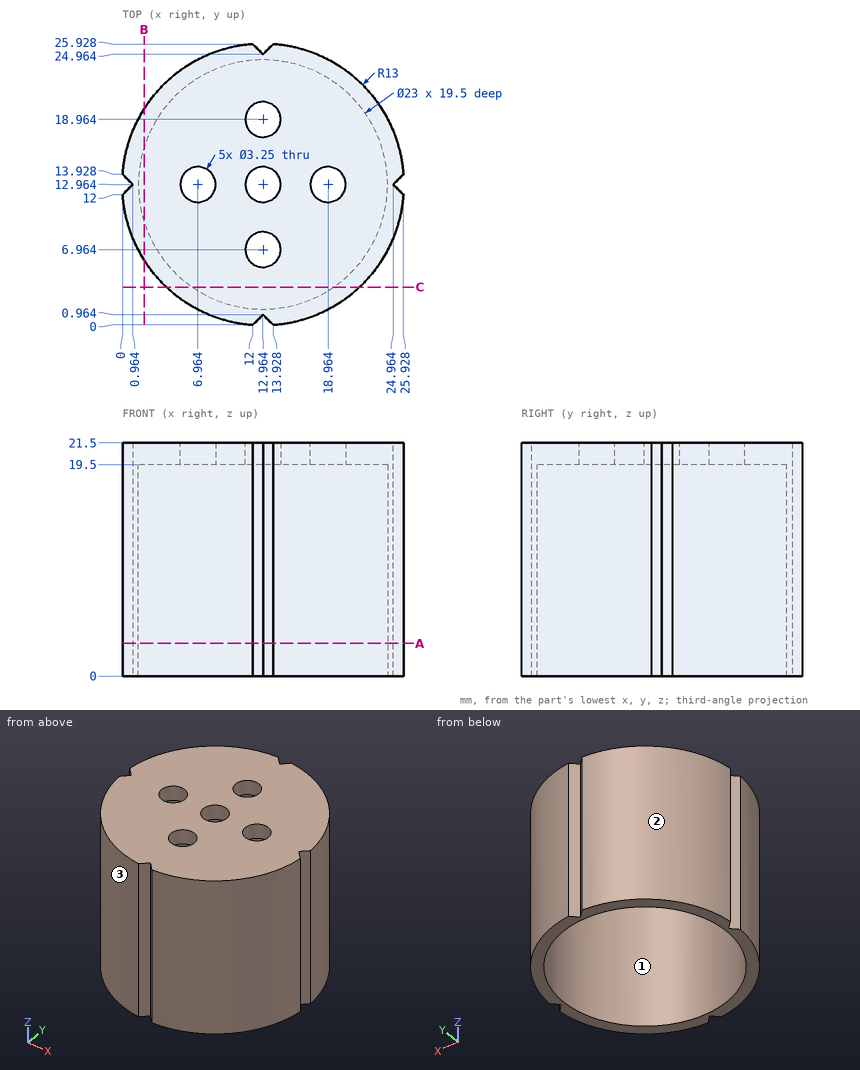
Study the drawing (mm; zero at the part's minimum x, y, z) and answer. Coordinates: 2 decimals unless noted, no trailing zeros. Write each loop counter-clockwise with the first axis right and the second up, starting at its lowest first coordinate (ties: lowest second). Pieces come first, ordered by that corner, then holes. Notation, with made-up numbers: (59.25, -18.75) - (110.25, -18.75) arc R12 ccw to (110.25, -8.75) - close; hole circle Ø11 at (65, -21). An arc over 180 degrees is marked (long way). Put each result on its own line as item: value.
1. The part is cut by section A-A on z = 3. Give the vertices of the cut face in (x, y).
Answer sheet:
outline: (0, 12) arc R13 ccw to (12, 0) - (12.96, 0.96) - (13.93, 0) arc R13 ccw to (25.93, 12) - (24.96, 12.96) - (25.93, 13.93) arc R13 ccw to (13.93, 25.93) - (12.96, 24.96) - (12, 25.93) arc R13 ccw to (0, 13.93) - (0.96, 12.96) - close; hole circle Ø23 at (12.96, 12.96)
2. Flat-ended cylindrical pins translate along their axes: pin 1 Ø12 at (x, z) = (22, 3) entering from +Y (1 decimal); pin 2 Ø3 at (y, z) = (8, 11.5) entering from +X; pin 3 Ø4 at (x, y) = (12.96, 12.96) entering from +Z; pin 4 Ø2.5 at (x, y) = (12.96, 6.96) entering from -Z. Find the tip coordinate at first contact, or state that the pin passes through.
Answer sheet:
pin 1: stops at y = 25.6
pin 2: stops at x = 25.49
pin 3: stops at z = 21.5
pin 4: passes through
3. The part is cut by section B-B on x = 2. Give the vertices of the cut face in (y, z) (1 decimal), plus the area to 3 significant figures.
Answer sheet:
outline: (6, 0) - (9.5, 0) - (9.5, 19.5) - (16.4, 19.5) - (16.4, 0) - (19.9, 0) - (19.9, 21.5) - (6, 21.5) - close
area: 165 mm^2
4. The part is cut by section C-C on y = 3.5. Give the vertices of the cut face in (x, z).
Answer sheet:
outline: (4.05, 0) - (6.43, 0) - (6.43, 19.5) - (19.5, 19.5) - (19.5, 0) - (21.88, 0) - (21.88, 21.5) - (4.05, 21.5) - close
5. Find the intervals of material crossed by line 1 along Z through (x, y) = (16.5, 17.75); line 2 along Y through (x, z) = (13, 16) (1 decimal); line 3 along Y through (x, z) = (9.5, 15.5) (1 decimal), in increasing order. Write a range as from..to.
Answer sheet:
line 1: z = 19.5..21.5
line 2: y = 0.9..1.5, 24.5..25
line 3: y = 0.4..2, 23.9..25.5
6. Determine the mould class of the marked faces 1, 2 and 3 for opening direction Y: pulls with the +Y half, pulls with the -Y half, needs draft (parallel to the pull), parting line crosses it, or undercut.
Answer sheet:
face 1: undercut
face 2: pulls with the +Y half
face 3: pulls with the -Y half
